Part model, mm, in its own coordinate system. Face numbers are marked on the shaded views. A direction names the side the tool comes from. Coordinates: 2 decimals unless noted, no trailing zeros. Loops run counter-clockwise (first coordinate to the right, second up) from the corner with the lowest first, then second, coordinate; pieces in that order, holes last. Notation, with made-up numbers: (51.5, 72.25) - (60.5, 72.25) arc R23 ccw to (60.5, 87.25) - close; hole circle Ø5 at (-35, -29.5). An arc over 180 degrees is marked (long way). One line per question, with ' | ' between items. Start each with the question number.
from build123d import *

# Parameters (mm, degrees)
SKETCH2_R           = 101.6
BOSS_EXTRUDE1_DEPTH = 50.8
SKETCH3_R           = 95.25
SKETCH3_R_2         = 19.685
CUT_EXTRUDE1_DEPTH  = 45.72
SKETCH4_R           = 17.272
CUT_EXTRUDE2_DEPTH  = 153.4
CUT_EXTRUDE3_START  = -19.05
CUT_EXTRUDE3_DEPTH  = 19.05
CIRPATTERN1_COUNT   = 8
WRAP1_START         = 2.54
WRAP1_DEPTH         = 25.4
CIRPATTERN2_COUNT   = 10
SKETCH9_R           = 3.175
CUT_EXTRUDE5_DEPTH  = 170.748495522
FILLET1_R           = 6.35


# Read off the part's stored shape, not the designer's step: Wrap1
with BuildPart() as part:
    # Sketch2 → Boss-Extrude1 (new body)
    with BuildSketch(Plane(origin=(0, 0, 0), x_dir=(1, 0, 0), z_dir=(0, 1, 0))):
        with Locations(Location((0, 0, 0), (0, 0, 270))):
            Circle(SKETCH2_R)
    extrude(amount=BOSS_EXTRUDE1_DEPTH)

    # Sketch3 → Cut-Extrude1 (cut)
    with BuildSketch(Plane(origin=(0, 50.8, 0), x_dir=(1, 0, 0), z_dir=(0, 1, 0))):
        with Locations(Location((0, 0, 0), (0, 0, 270))):
            Circle(SKETCH3_R)
        with Locations(Location((0, 0, 0), (0, 0, 270))):
            Circle(SKETCH3_R_2, mode=Mode.SUBTRACT)
    extrude(amount=-CUT_EXTRUDE1_DEPTH, mode=Mode.SUBTRACT)

    # Sketch4 → Cut-Extrude2 (cut, through all)
    with BuildSketch(Plane(origin=(0, 50.8, 0), x_dir=(1, 0, 0), z_dir=(0, 1, 0))):
        with Locations(Location((0, 0, 0), (0, 0, 270))):
            Circle(SKETCH4_R)
    extrude(amount=-CUT_EXTRUDE2_DEPTH, mode=Mode.SUBTRACT)

    # Sketch5 → Cut-Extrude3 (cut)
    with BuildSketch(Plane(origin=(0, 50.8, 0), x_dir=(1, 0, 0), z_dir=(0, 1, 0)).offset(CUT_EXTRUDE3_START)):
        with BuildLine():
            Line((0, 101.6), (0, 94.154505037))
            ThreePointArc((0, 94.154505037), (16.351324372, 92.723810373), (32.205726105, 88.475205707))
            Line((32.205726105, 88.475205707), (34.752471706, 95.471596354))
            ThreePointArc((34.752471706, 95.471596354), (17.644344851, 100.056169699), (0, 101.6))
        make_face()
    cut_extrude3 = extrude(amount=CUT_EXTRUDE3_DEPTH, mode=Mode.SUBTRACT)

    # CirPattern1: Cut-Extrude3 ×8 about axis
    cirpattern1_axis = Axis((0, 0, 0), (0, 1, 0))
    for i in range(1, CIRPATTERN1_COUNT):
        add(cut_extrude3.rotate(cirpattern1_axis, i * 360 / CIRPATTERN1_COUNT), mode=Mode.SUBTRACT)

    # Wrap1 outline → Wrap1 (add)
    with BuildSketch(Plane(origin=(0, 0, 0), x_dir=(1, 0, 0), z_dir=(0, 1, 0)).offset(WRAP1_START)):
        with BuildLine():
            ThreePointArc((98.742950455, -28.845565264), (102.869546579, -0.305428593), (98.912497991, 28.258709119))
            Line((98.912497991, 28.258709119), (97.691356041, 27.909836167))
            ThreePointArc((97.691356041, 27.909836167), (101.599552177, -0.30165787), (97.523901684, -28.489447175))
            Line((97.523901684, -28.489447175), (98.742950455, -28.845565264))
        make_face()
    wrap1 = extrude(amount=WRAP1_DEPTH)

    # CirPattern2: Wrap1 ×10 about axis
    cirpattern2_axis = Axis((0, 0, 0), (0, 1, 0))
    for i in range(1, CIRPATTERN2_COUNT):
        add(wrap1.rotate(cirpattern2_axis, i * 360 / CIRPATTERN2_COUNT))

    # Sketch9 → Cut-Extrude5 (cut, through all)
    with BuildSketch(Plane(origin=(19.385940618, 0, 3.418264377), x_dir=(0, 1, 0), z_dir=(0.9848077530122106, 0, 0.17364817766691706))):
        with Locations(Location((38.1, 0, 0), (0, 0, 270))):
            Circle(SKETCH9_R)
    extrude(amount=-CUT_EXTRUDE5_DEPTH, mode=Mode.SUBTRACT)

    # Fillet1
    fillet1_edges = [part.edges().sort_by_distance(p)[0] for p in [
        (0, 5.08, -19.685),
    ]]
    fillet(fillet1_edges, radius=FILLET1_R)


solid = part.part
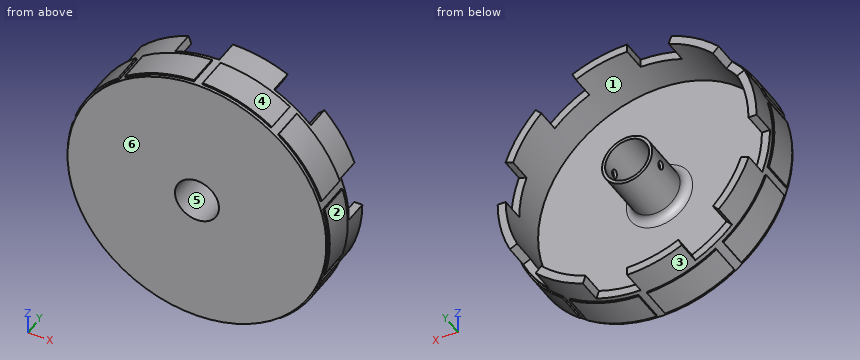
1) Tool access for the marked faces 1, 2 and 3: list every direction of +Z, -Z, +X, -X, +Y, -Y with a clear straight run to the whole face (end or side of a thin tool).
2) Pin check, flat tips, straight feed: pin 1 Ø3 at (y, z) = (13.5, 73) entering from +X; pin 2 Ø10 at (y, z) = (28, -9.5) entering from -X; pin 3 Ø6 at (x, z) = (-94, -11) entering from +Y. Stop position of each tip, or through.
3) Wall check: line 1 along X through (y, z) = (26.5, 0) (3 decimals); line 2 along X through (y, z) = (29, 0) (3 decimals); line 3 along X through (y, z) = (44, 2). Give the ranges that are in metal, low to high. Write a range as [from, to].
4) Band-saw the part on B-B on x = 76.5. List the corners of the cut face in (y, z), then the cut area to 3 significant figures.
5) Band-saw the part on C-C on y = 8.5. Count the separate pieces of the cut face and the enclosed holes in it, then the cut area to 3 significant figures.
6) Mould opens along X. For the marked faces 4, 5 and 6 say: +X half, -X half, draft (parallel to the pull), parting line (faces both ways), or undercut.
7) Band-saw the part on A-A on z = -53. List the corners of the cut face in (x, y).
Values found:
1) face 1: +Y | face 2: +X, +Y, -Y | face 3: none
2) pin 1: x = 73.96 | pin 2: x = -102.77 | pin 3: y = 31.75
3) line 1: [-102.87, -95.25], [-19.685, -17.272], [17.272, 19.685], [95.25, 102.87] | line 2: [-101.6, -95.25], [-19.685, -17.272], [17.272, 19.685], [95.25, 101.6] | line 3: [-101.58, -95.23], [-19.58, -17.16], [17.16, 19.58]
4) outline: (0, -66.86) - (2.54, -66.86) - (2.54, -68.77) - (27.94, -68.77) - (27.94, -66.86) - (31.75, -66.86) - (31.75, -56.75) - (5.08, -56.75) - (5.08, 56.75) - (50.8, 56.75) - (50.8, 66.86) - (27.94, 66.86) - (27.94, 68.77) - (2.54, 68.77) - (2.54, 66.86) - (0, 66.86) - close | area: 1,510 mm²
5) separate pieces: 2 | enclosed holes: 2 | area: 5,030 mm²
6) face 4: +X half | face 5: undercut | face 6: draft
7) outline: (-88.17, 2.54) - (-86.68, 2.54) - (-86.68, 0) - (86.68, 0) - (86.68, 2.54) - (88.17, 2.54) - (88.17, 27.94) - (86.68, 27.94) - (86.68, 31.75) - (79.14, 31.75) - (79.14, 5.08) - (-79.14, 5.08) - (-79.14, 50.8) - (-86.68, 50.8) - (-86.68, 27.94) - (-88.17, 27.94) - close
